```python
from build123d import *

# Parameters (mm, degrees)
SKETCH1_W           = 107.786447668
SKETCH1_H           = 124.928058302
SKETCH1_R           = 1.5748
BOSS_EXTRUDE1_DEPTH = 1.5875
FILLET1_R           = 5.08
CUT_EXTRUDE1_DEPTH  = 83.515178417
SKETCH6_W           = 95.25
SKETCH6_H           = 111.125
BOSS_EXTRUDE2_DEPTH = 0.396875


with BuildPart() as part:
    # Sketch1 → Boss-Extrude1 (new body)
    with BuildSketch(Plane.XY):
        Rectangle(SKETCH1_W, SKETCH1_H)
        with Locations((-49.911, 57.8485)):
            Circle(SKETCH1_R, mode=Mode.SUBTRACT)
        with Locations((49.911, 57.8485)):
            Circle(SKETCH1_R, mode=Mode.SUBTRACT)
        with Locations((49.911, -57.8485)):
            Circle(SKETCH1_R, mode=Mode.SUBTRACT)
        with Locations((-49.911, -57.8485)):
            Circle(SKETCH1_R, mode=Mode.SUBTRACT)
    extrude(amount=BOSS_EXTRUDE1_DEPTH)

    # Fillet1
    fillet1_edges = [part.edges().sort_by_distance(p)[0] for p in [
        (-53.893223834, 62.464029151, 0.79375),
        (53.893223834, 62.464029151, 0.79375),
        (53.893223834, -62.464029151, 0.79375),
        (-53.893223834, -62.464029151, 0.79375),
    ]]
    fillet(fillet1_edges, radius=FILLET1_R)

    # Sketch4 → Cut-Extrude1 (cut, through all)
    with BuildSketch(Plane.XY.offset(1.5875)):
        with BuildLine():
            Line((41.275, 55.5625), (-41.275, 55.5625))
            ThreePointArc((-41.275, 55.5625), (-45.765128061, 53.702628061), (-47.625, 49.2125))
            Line((-47.625, 49.2125), (-47.625, -49.2125))
            ThreePointArc((-47.625, -49.2125), (-45.765128061, -53.702628061), (-41.275, -55.5625))
            Line((-41.275, -55.5625), (41.275, -55.5625))
            ThreePointArc((41.275, -55.5625), (45.765128061, -53.702628061), (47.625, -49.2125))
            Line((47.625, -49.2125), (47.625, 49.2125))
            ThreePointArc((47.625, 49.2125), (45.765128061, 53.702628061), (41.275, 55.5625))
        make_face()
    extrude(amount=-CUT_EXTRUDE1_DEPTH, mode=Mode.SUBTRACT)

    # Sketch6 → Boss-Extrude2 (add)
    with BuildSketch(Plane(origin=(0, 0, 0), x_dir=(-1, 0, 0), z_dir=(0, 0, -1))):
        Rectangle(SKETCH6_W, SKETCH6_H)
    extrude(amount=-BOSS_EXTRUDE2_DEPTH)


solid = part.part
```
Source: CAD feature listing. Evaluate the final solid. Frame: model axes, mm. A direction names the side the tool comes from. Give positions to 0.01 mm unless a question says otherwise; leave off trailing zeros. Loops run counter-clockwise (first coordinate to the right, second up) from the corner with the lowest first, then second, coordinate; pieces in that order, holes last. Notation, with made-up numbers: (27, 46) - (75, 46) arc R13 cw to (75, 61) - close; hole circle Ø10 at (47.25, 20.5). An arc over 180 degrees is marked (long way). Use CSV: the item, a comma, the result in double quotes.
1) Set-up query: faces 1 (the cylindrical face through (45.814, 53.653, 1.001)), 2 (the cylindrical face through (49.57, -59.386, 0.783)). Return all of +Z, -Z, +X, -X, +Y, -Y with unobstructed straight access to the full face (end or side cutting, diameter ignored); none if empty.
Worked out:
face 1,"+Z"
face 2,"+Z, -Z"
2) Pin query (flat end, axial travel): P1, Ø3, axis at x = 17, y = 33.5, coming from the +Z side; P2, Ø3, axis at x = 49.91, y = -57.85, coming from the -Z side. Return the tip coordinate at first contact, or that it passes through.
Worked out:
P1,"stops at z = 0.4"
P2,"passes through"
3) Cut plane B-B (z = 1.2). Count the separate pieces of the cut face and the enclosed holes in it, and give its area (3 significant figures).
Worked out:
separate pieces,"1"
enclosed holes,"5"
area,"2,860 mm^2"
4) Mould query, pull axis X, two halves, no side actions, for faces 3 (the cylindrical face through (52.366, 61.015, 0.805)), 4 (the cylindrical face through (-49.184, -59.246, 0.783)), 5 (the flat face through (48, 10, 1.588)). Classes: +X half, -X half, draft (parallel to the pull), parting line (faces both ways), or undercut.
Worked out:
face 3,"+X half"
face 4,"undercut"
face 5,"draft"
5) Cut plane C-C (y = 0). Output: boundary loops of the cut face in (x, z) (1 decimal), and give its area (3 significant figures).
Worked out:
outline,"(-53.9, 0) - (53.9, 0) - (53.9, 1.6) - (47.6, 1.6) - (47.6, 0.4) - (-47.6, 0.4) - (-47.6, 1.6) - (-53.9, 1.6) - close"
area,"57.7 mm^2"
6) Line query: line 1 (X direction, y = 21.5, z = 0.55) (3 decimals); line 2 (Y direction, x = -35, z = 0.5); line 3 (X direction, y = 57, z = 1.15). Output: solid intervals per line, ascending.
Worked out:
line 1,"x = -53.893 to -47.625, 47.625 to 53.893"
line 2,"y = -62.46 to -55.56, 55.56 to 62.46"
line 3,"x = -53.89 to -51.24, -48.58 to 48.58, 51.24 to 53.89"
7) Cut plane A-A (x = -2). Output: boundary loops of the cut face in (y, z).
Worked out:
outline,"(-62.46, 0) - (62.46, 0) - (62.46, 1.59) - (55.56, 1.59) - (55.56, 0.4) - (-55.56, 0.4) - (-55.56, 1.59) - (-62.46, 1.59) - close"
